Build history of the part. All positions in model axes, mm. A direction names the side the tool comes from. Round coordinates to 2 decimals unless told otherwise and drop trailing zeros. Order: outer loops, then holes, each group sorted by start corner. A loop starts at its lowest first (then second) coordinate and runs counter-clockwise, first axis right, second up. Notation, with made-up numbers: (52, -5.75) -> (103, -5.75) arc R15 cw to (103, 13.25) -> close; hole circle Ø4 at (-15, 68). An arc over 180 degrees is marked (long way). Answer as a JSON object with one key per item and string values.
from build123d import *

# Parameters (mm, degrees)
F0_R     = 12
F0_R_2   = 14.5
F0_R_3   = 11
F1_DEPTH = 7


with BuildPart() as f1:
    # F0 (on Top) → F1 (new body)
    with BuildSketch(Plane.XY):
        with BuildLine():
            ThreePointArc((13.007052, 26.028949), (14.493201, 29.63385), (15, 33.5))
            ThreePointArc((15, 33.5), (-3.86615, 47.993201), (-13.007052, 26.028949))
            ThreePointArc((-13.007052, 26.028949), (0, 18.5), (13.007052, 26.028949))
        make_face()
        with Locations((0, 33.5)):
            Circle(F0_R, mode=Mode.SUBTRACT)
        with BuildLine():
            ThreePointArc((13.007052, 26.028949), (0, 18.5), (-13.007052, 26.028949))
            ThreePointArc((-13.007052, 26.028949), (-10.880101, 16.688967), (-12.577073, 7.261376))
            ThreePointArc((-12.577073, 7.261376), (-19.89312, 1.07796), (-29.045257, -1.750037))
            ThreePointArc((-29.045257, -1.750037), (-18.417067, -6.131594), (-14.011851, -16.75))
            ThreePointArc((-14.011851, -16.75), (-14.527296, -20.648417), (-16.038205, -24.278912))
            ThreePointArc((-16.038205, -24.278912), (-9.013019, -17.766927), (0, -14.522753))
            ThreePointArc((0, -14.522753), (9.013019, -17.766927), (16.038205, -24.278912))
            ThreePointArc((16.038205, -24.278912), (16.02147, -9.25), (29.045257, -1.750037))
            ThreePointArc((29.045257, -1.750037), (19.89312, 1.07796), (12.577073, 7.261376))
            ThreePointArc((12.577073, 7.261376), (10.880101, 16.688967), (13.007052, 26.028949))
        make_face()
        Circle(F0_R_2, mode=Mode.SUBTRACT)
        with BuildLine():
            ThreePointArc((-14.011851, -16.75), (-18.417067, -6.131594), (-29.045257, -1.750037))
            ThreePointArc((-29.045257, -1.750037), (-42.002232, -24.25), (-16.038205, -24.278912))
            ThreePointArc((-16.038205, -24.278912), (-14.527296, -20.648417), (-14.011851, -16.75))
        make_face()
        with Locations((-29.011851, -16.75)):
            Circle(F0_R, mode=Mode.SUBTRACT)
        with BuildLine():
            ThreePointArc((44.011851, -16.75), (39.630257, -6.155216), (29.045257, -1.750037))
            ThreePointArc((29.045257, -1.750037), (16.02147, -9.25), (16.038205, -24.278912))
            ThreePointArc((16.038205, -24.278912), (32.910268, -31.234555), (44.011851, -16.75))
        make_face()
        with Locations((29.011851, -16.75)):
            Circle(F0_R, mode=Mode.SUBTRACT)
        Circle(F0_R_2)
        Circle(F0_R_3, mode=Mode.SUBTRACT)
    extrude(amount=F1_DEPTH)


solid = f1.part
1) Flat gauge pins, fed straight in: pin 1 Ø2 at (y, z) = (-8, 3) entering from +X; pin 2 Ø1 at (x, z) = (-18.5, 3.5) entering from +Y; pin 3 Ø4 at (x, z) = (27.5, 3.5) entering from -Y; pin 4 Ø4 at (y, z) = (-11.5, 1) entering from +X. Where does each tip first touch, or does it go through?
Checked values:
{"pin 1": "stops at x = 41.85", "pin 2": "stops at y = 2.23", "pin 3": "stops at y = -31.75", "pin 4": "stops at x = 43.66"}
2) Pull direction Y, two halves, no side cores. Call faces 4 (the face through (-9.13, -17.84, 3.45)), 5 (the face through (14.48, 29.58, 3.45)), 6 (the face through (-42.2, -23.9, 3.5)), 7 (the face through (6.3, -9.3, 7)): pulls with the +Y half, pulls with the -Y half, needs draft (parallel to the pull), parting line crosses it, or undercut.
Checked values:
{"face 4": "pulls with the -Y half", "face 5": "undercut", "face 6": "parting line crosses it", "face 7": "needs draft"}
3) Probe L1, parallel to Y at x = 0, z = 4.25; L2, parallel to Y at x = -6.5, z = 2.25; L3, parallel to X at y = -12, z = 0.75. List the from-to ranges inside material, lowest first. Write a range as from..to.
Checked values:
{"L1": "y = -14.52..-11, 11..21.5, 45.5..48.5", "L2": "y = -16.44..-8.87, 8.87..23.41, 43.59..47.02", "L3": "x = -43.24..-40.03, -17.99..17.99, 40.03..43.24"}
4) Cut at C-C, the plane x = 30. Give the cut face in (y, z).
Checked values:
{"outline": "(-31.72, 0) -> (-28.71, 0) -> (-28.71, 7) -> (-31.72, 7) -> close; (-4.79, 0) -> (-1.78, 0) -> (-1.78, 7) -> (-4.79, 7) -> close"}
5) Cut at D-D, the plane x = -7. Give the cut face in (y, z), plus the area to 3 significant figures.
Checked values:
{"outline": "(-16.67, 0) -> (-8.49, 0) -> (-8.49, 7) -> (-16.67, 7) -> close; (8.49, 0) -> (23.75, 0) -> (23.75, 7) -> (8.49, 7) -> close; (43.25, 0) -> (46.77, 0) -> (46.77, 7) -> (43.25, 7) -> close", "area": "189 mm²"}
6) Cut at B-B, the plane y = 4.5. Give the cut face in (x, z).
Checked values:
{"outline": "(-15.13, 0) -> (-10.04, 0) -> (-10.04, 7) -> (-15.13, 7) -> close; (10.04, 0) -> (15.13, 0) -> (15.13, 7) -> (10.04, 7) -> close"}
7) Cut at A-A, the plane z = 5.75. Give the cut face in (x, y), plus the area to 3 significant figures.
Checked values:
{"outline": "(-29.05, -1.75) arc R15 ccw (long way) to (-16.04, -24.28) arc R23.99 cw to (0, -14.52) arc R23.99 cw to (16.04, -24.28) arc R15 ccw to (44.01, -16.75) arc R15 ccw to (29.05, -1.75) arc R23.99 cw to (12.58, 7.26) arc R23.99 cw to (13.01, 26.03) arc R15 ccw to (15, 33.5) arc R15 ccw (long way) to (-13.01, 26.03) arc R23.99 cw to (-12.58, 7.26) arc R23.99 cw to start; hole circle Ø24 at (-29.01, -16.75); hole circle Ø24 at (0, 33.5); hole circle Ø22 at (0, 0); hole circle Ø24 at (29.01, -16.75)", "area": "1,540 mm²"}
8) Which spindle directions (+Z, -Z, +X, -X, +Y, -Y) get a long thin tool onto all of the face, cutting with end or side? Do faces 1 (the face through (-19.775, 1.143, 3.451)), 2 (the face through (8.9, -17.7, 3.5)), 3 (the face through (20.012, 1.013, 3.451)). Say none if no direction does.
Checked values:
{"face 1": "+Z, -Z, -X", "face 2": "+Z, -Z, -Y", "face 3": "+Z, -Z, +X"}
